Read the model definition and answer for the solid it produces. Units are mm, in the model's axes. A direction names the side the tool comes from. Coordinates: 2 decimals unless noted, no trailing zeros. Order: outer loops, then holes, each group sorted by start corner. A loop starts at its lowest first (then second) coordinate and runs counter-clockwise, first axis right, second up. Notation, with made-up numbers: M 88.5,-5 L 112.5,-5 A29 ccw 112.5,17 Z; hole C -1.5,51.25 d7. An arc over 180 degrees is marked long. Use a Markdown table: item, result. Add a question column.
1) The mould has two halves that part along Z. Classify faces 1 (the face through (20, 0, 23)), 2 (the face through (9.67, 2.54, 22.52)), 3 (the face through (20.28, 5.6, 5.57)), 4 (the face through (20.28, 1.88, 1.78)): released by +Z, released by -Z, zero draft, split by the parting line, or undercut.
2) Find section D-D on x = 30. Write down the section's boundary in (y, z).
3) Find the intervals of material crossed by probe 1 along X at (y, z) = (1.9, 25); probe 2 along Y at (x, z) = (30.5, 11.5), in increasing order. Write a range as [from, to].
4) Find section A-A on x = 20. Write down the section's boundary in (y, z), plus the area to 3 significant figures.
5) Find section C-C on x = 34.5. Write down the section's boundary in (y, z).
6) Find section B-B on y = 22. Write down the section's boundary in (x, z).
7) Each of these flat-tipped pins is pushed along its axis until it touches: pin 1 Ø4 at (x, z) = (25, 8.5) entering from +Y; pin 2 Ø4 at (x, z) = (30, 25) entering from -Y; pin 3 Ø5 at (x, y) = (4, 30.5) entering from +Z; pin 4 Ø16.5 at (x, z) = (17, 18) entering from +Y. Where does it stop, or does it pass through?
8) For faces 5 (the face through (18.92, 20.12, 2.54)), 6 (the face through (20, 5, 23)), determine the directions among +Z, -Z, +X, -X, +Y, -Y from which every point of the face is accessible in a straight line to the end or side of a thin tool.
from build123d import *

# Parameters (mm, degrees)
SKETCH2_W           = 40
SKETCH2_H           = 5
BOSS_EXTRUDE1_DEPTH = 40
SKETCH3_W           = 40
SKETCH3_H           = 5
BOSS_EXTRUDE2_DEPTH = 40
SKETCH4_R           = 2.5
CUT_EXTRUDE1_DEPTH  = 10
SKETCH5_R           = 5
CUT_EXTRUDE2_DEPTH  = 10
FILLET1_R           = 6.25
FILLET2_R           = 2


with BuildPart() as part:
    # Sketch2 → Boss-Extrude1 (new body)
    with BuildSketch(Plane.XY):
        with Locations((20, 2.5)):
            Rectangle(SKETCH2_W, SKETCH2_H)
    extrude(amount=BOSS_EXTRUDE1_DEPTH)

    # Sketch3 → Boss-Extrude2 (add)
    with BuildSketch(Plane(origin=(0, 5, 0), x_dir=(1, 0, 0), z_dir=(0, 1, 0))):
        with Locations((20, -2.5)):
            Rectangle(SKETCH3_W, SKETCH3_H)
    extrude(amount=BOSS_EXTRUDE2_DEPTH)

    # Sketch4 → Cut-Extrude1 (cut)
    with BuildSketch(Plane(origin=(0, 5, 0), x_dir=(1, 0, 0), z_dir=(0, 1, 0))):
        with Locations((10, -25)):
            Circle(SKETCH4_R)
        with Locations((30, -25)):
            Circle(SKETCH4_R)
    extrude(amount=-CUT_EXTRUDE1_DEPTH, mode=Mode.SUBTRACT)

    # Sketch5 → Cut-Extrude2 (cut)
    with BuildSketch(Plane.XY.offset(5)):
        with Locations((20, 25)):
            Circle(SKETCH5_R)
    extrude(amount=-CUT_EXTRUDE2_DEPTH, mode=Mode.SUBTRACT)

    # Fillet1
    fillet1_edges = [part.edges().sort_by_distance(p)[0] for p in [
        (20, 0, 0),
    ]]
    fillet(fillet1_edges, radius=FILLET1_R)

    # Fillet2
    fillet2_edges = [part.edges().sort_by_distance(p)[0] for p in [
        (20, 5, 5),
    ]]
    fillet(fillet2_edges, radius=FILLET2_R)


solid = part.part
Check result:
| question | item | result |
|---|---|---|
| 1 | face 1 | zero draft |
| 1 | face 2 | undercut |
| 1 | face 3 | released by +Z |
| 1 | face 4 | released by -Z |
| 2 | outline | M 0,6.25 A6.25 ccw 6.25,0 L 45,0 L 45,5 L 7,5 A2 cw 5,7 L 5,22.5 L 0,22.5 Z; M 0,27.5 L 5,27.5 L 5,40 L 0,40 Z |
| 3 | probe 1 | x = [0, 7.5], [12.5, 27.5], [32.5, 40] |
| 3 | probe 2 | y = [0, 5] |
| 4 | outline | M 0,6.25 A6.25 ccw 6.25,0 L 20,0 L 20,5 L 7,5 A2 cw 5,7 L 5,40 L 0,40 Z; M 30,0 L 45,0 L 45,5 L 30,5 Z |
| 4 | area | 342 mm2 |
| 5 | outline | M 0,6.25 A6.25 ccw 6.25,0 L 45,0 L 45,5 L 7,5 A2 cw 5,7 L 5,40 L 0,40 Z |
| 6 | outline | M 0,0 L 16,0 L 16,5 L 0,5 Z; M 24,0 L 40,0 L 40,5 L 24,5 Z |
| 7 | pin 1 | stops at y = 5.06 |
| 7 | pin 2 | passes through |
| 7 | pin 3 | stops at z = 5 |
| 7 | pin 4 | stops at y = 5 |
| 8 | face 5 | +Z, -Z |
| 8 | face 6 | +Z, +X, -X, +Y |
